```python
from build123d import *

# Parameters (mm, degrees)
F1_DEPTH = 215.9
F0_W     = 73.025
F0_H     = 82.55
F2_DEPTH = 25.4
F4_DEPTH = 120.65
F5_DEPTH = 127
F6_DEPTH = 6.35


with BuildPart() as f1:
    # F0 (on Top) → F1 (new body)
    with BuildSketch(Plane.XY):
        Polygon((73.025, 82.55), (73.025, 0), (92.075, 0), (92.075, 82.55), (165.1, 82.55), (165.1, 101.6), (0, 101.6), (0, 82.55), align=None)
    extrude(amount=F1_DEPTH)

    # F0 (on Top) + F1_face (on face) → F2 (join)
    with BuildSketch(Plane.XY):
        with Locations((36.5125, 41.275)):
            Rectangle(F0_W, F0_H)
        with Locations((128.5875, 41.275)):
            Rectangle(F0_W, F0_H)
    with BuildSketch(Plane(origin=(82.55, 75.141667, 215.9), x_dir=(1, 0, 0), z_dir=(0, 0, 1))):
        Polygon((-9.525, 7.408333), (-9.525, -75.141667), (9.525, -75.141667), (9.525, 7.408333), (82.55, 7.408333), (82.55, 26.458333), (-82.55, 26.458333), (-82.55, 7.408333), align=None)
    extrude(amount=F2_DEPTH)

    # F3 (on face) → F4 (join)
    with BuildSketch(Plane(origin=(0, 101.6, 0), x_dir=(-1, 0, 0), z_dir=(0, 1, 0))):
        with BuildLine():
            Line((-133.35, 241.3), (-146.05, 241.3))
            ThreePointArc((-146.05, 241.3), (-82.55, 177.8), (-19.05, 241.3))
            Line((-19.05, 241.3), (-31.75, 241.3))
            Line((-31.75, 241.3), (-31.75, 234.95))
            Line((-31.75, 234.95), (-44.982893, 234.95))
            ThreePointArc((-44.982893, 234.95), (-82.55, 203.2), (-120.117107, 234.95))
            Line((-120.117107, 234.95), (-133.35, 234.95))
            Line((-133.35, 234.95), (-133.35, 241.3))
        make_face()
    extrude(amount=-F4_DEPTH)

    # F3 (on face) → F5 (cut)
    with BuildSketch(Plane(origin=(0, 101.6, 0), x_dir=(-1, 0, 0), z_dir=(0, 1, 0))):
        with BuildLine():
            Line((-82.55, 241.3), (-133.35, 241.3))
            Line((-133.35, 241.3), (-133.35, 234.95))
            Line((-133.35, 234.95), (-120.117107, 234.95))
            ThreePointArc((-120.117107, 234.95), (-82.55, 203.2), (-44.982893, 234.95))
            Line((-44.982893, 234.95), (-31.75, 234.95))
            Line((-31.75, 234.95), (-31.75, 241.3))
            Line((-31.75, 241.3), (-82.55, 241.3))
        make_face()
    extrude(amount=-F5_DEPTH, mode=Mode.SUBTRACT)

    # F3 (on face) → F6 (join)
    with BuildSketch(Plane(origin=(0, 101.6, 0), x_dir=(-1, 0, 0), z_dir=(0, 1, 0))):
        with BuildLine():
            Line((-133.35, 241.3), (-146.05, 241.3))
            ThreePointArc((-146.05, 241.3), (-82.55, 177.8), (-19.05, 241.3))
            Line((-19.05, 241.3), (-31.75, 241.3))
            Line((-31.75, 241.3), (-31.75, 234.95))
            Line((-31.75, 234.95), (-44.982893, 234.95))
            ThreePointArc((-44.982893, 234.95), (-82.55, 203.2), (-120.117107, 234.95))
            Line((-120.117107, 234.95), (-133.35, 234.95))
            Line((-133.35, 234.95), (-133.35, 241.3))
        make_face()
    extrude(amount=F6_DEPTH)


solid = f1.part
```
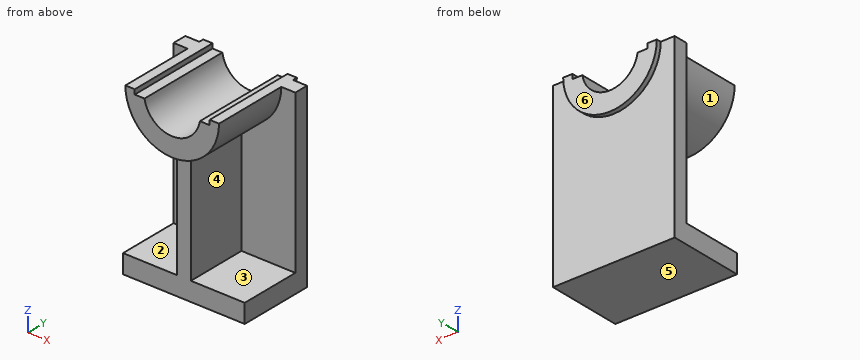
Design review of the part built by this model. Coordinates are the model's own, in mm. Face numbers are marked on the shaded views. A direction names the side the tool comes from. Give positions to 0.01 mm unless a question says otherwise; leave off trailing zeros. Order: outer loops, then holes, each group sorted by start corner. A loop starts at its lowest first (then second) coordinate and runs counter-clockwise, first axis right, second up. Notation, with made-up numbers: (46.25, 37.5) -> (101.25, 37.5) arc R5 cw to (101.25, 43.5) -> close; hole circle Ø1 at (-12.5, -5.5). An arc over 180 degrees is marked (long way). Write each question's results on one line, items separated by ' | '. Start each with the question number.
Q1. Add section C-C on z = 210.5. Give the boundary of the cut face in (x, y).
Q2. Add section A-A on x = 82.55. Give the boundary of the cut face in (y, z).
Q3. Add section B-B on y = 75. Give the boundary of the cut face in (x, z) (3 decimals), and give its area (3 significant figures).
Q4. Wall thickness on L1, parallel to Y at x = 117, z = 143; L2, parallel to Z at x = 56, y = 43; L3, parallel to Z at x = 84, y = 80: over which ranges is each line inside the solid? List them lowest first. Write a range as from..to.
Q5. Mouldability with a two-part tool opening along Z and no side actions: class the marked faces 4, 5 and 6 as +Z half, -Z half, draft (parallel to the pull), parting line (faces both ways), or undercut.
Q6. Machinability: for the marked faces 1, 2 and 3, which of the approach directions +Z, -Z, +X, -X, +Y, -Y give a long, thin tool a straight path to every point of the face, cutting with its end or side? Answer none if there is none.
Q7. Add section D-D on x = 40. Give the boundary of the cut face in (y, z), and give its area (3 significant figures).
Q8. For pin 1 (5 mm diameter, centred on y = 64, z = 237, fed in from -X); pin 2 (1.9 mm diameter, centred on y = 51, z = 239, fed in from +X); pin 3 (2 mm diameter, centred on x = 64.5, z = 31.5, fed in from +Y), all flat-tipped, find the tip position at first contact; note any pin that passes through.
Found:
1) outline: (0, 82.55) -> (27.02, 82.55) -> (27.02, -19.05) -> (60.12, -19.05) -> (60.12, 107.95) -> (27.02, 107.95) -> (27.02, 101.6) -> (0, 101.6) -> close; (104.98, -19.05) -> (138.08, -19.05) -> (138.08, 82.55) -> (165.1, 82.55) -> (165.1, 101.6) -> (138.08, 101.6) -> (138.08, 107.95) -> (104.98, 107.95) -> close
2) outline: (-19.05, 177.8) -> (0, 177.8) -> (0, 0) -> (101.6, 0) -> (101.6, 177.8) -> (107.95, 177.8) -> (107.95, 203.2) -> (-19.05, 203.2) -> close
3) outline: (0, 0) -> (165.1, 0) -> (165.1, 25.4) -> (92.075, 25.4) -> (92.075, 178.518) arc R63.5 ccw to (146.05, 241.3) -> (133.35, 241.3) -> (133.35, 234.95) -> (120.117, 234.95) arc R38.1 cw to (44.983, 234.95) -> (31.75, 234.95) -> (31.75, 241.3) -> (19.05, 241.3) arc R63.5 ccw to (73.025, 178.518) -> (73.025, 25.4) -> (0, 25.4) -> close | area: 11,000 mm2
4) L1: y = 82.55..101.6 | L2: z = 0..25.4, 183.62..213.97 | L3: z = 0..203.23
5) face 4: undercut | face 5: -Z half | face 6: draft
6) face 1: -Y | face 2: -X, -Y | face 3: +X, -Y
7) outline: (-19.05, 194.16) -> (82.55, 194.16) -> (82.55, 25.4) -> (0, 25.4) -> (0, 0) -> (101.6, 0) -> (101.6, 194.16) -> (107.95, 194.16) -> (107.95, 234.95) -> (-19.05, 234.95) -> close | area: 11,000 mm2
8) pin 1: stops at x = 19.08 | pin 2: stops at x = 146.04 | pin 3: stops at y = 101.6
